```python
from build123d import *

# Parameters (mm, degrees)
F1_DEPTH = 0.91
F3_DEPTH = 5.4
F4_R     = 2.375
F5_DEPTH = 1
F6_R     = 2.375
F7_DEPTH = 3
F9_D     = 2.5
F11_D    = 1


with BuildPart() as f1:
    # F0 (on Top) → F1 (new body, symmetric)
    with BuildSketch(Plane.XY):
        with BuildLine():
            Line((-13.92, -1.75), (-13.92, 1.75))
            ThreePointArc((-13.92, 1.75), (-15.67, 0), (-13.92, -1.75))
        make_face()
        with BuildLine():
            ThreePointArc((-13.92, 1.75), (-12.682563, 1.237437), (-12.17, 0))
            ThreePointArc((-12.17, 0), (-12.682563, -1.237437), (-13.92, -1.75))
            Line((-13.92, -1.75), (0, -2.45))
            Line((0, -2.45), (0, 2.45))
            Line((0, 2.45), (-13.92, 1.75))
        make_face()
        with BuildLine():
            ThreePointArc((-13.92, -1.75), (-12.682563, -1.237437), (-12.17, 0))
            ThreePointArc((-12.17, 0), (-12.682563, 1.237437), (-13.92, 1.75))
            Line((-13.92, 1.75), (-13.92, -1.75))
        make_face()
    extrude(amount=F1_DEPTH, both=True)

    # F2 (on face) → F3 (join)
    with BuildSketch(Plane.XY.offset(0.91)):
        with BuildLine():
            ThreePointArc((-2.509238, -2.323817), (1.24796, -3.184179), (3.42, 0))
            ThreePointArc((3.42, 0), (1.24796, 3.184179), (-2.509238, 2.323817))
            Line((-2.509238, 2.323817), (0, 2.45))
            Line((0, 2.45), (0, -2.45))
            Line((0, -2.45), (-2.509238, -2.323817))
        make_face()
        with BuildLine():
            Line((0, 2.45), (-2.509238, 2.323817))
            ThreePointArc((-2.509238, 2.323817), (-3.42, 0), (-2.509238, -2.323817))
            Line((-2.509238, -2.323817), (0, -2.45))
            Line((0, -2.45), (0, 2.45))
        make_face()
    extrude(amount=-F3_DEPTH)

    # F4 (on face) → F5 (cut)
    with BuildSketch(Plane.XY.offset(0.91)):
        Circle(F4_R)
    extrude(amount=-F5_DEPTH, mode=Mode.SUBTRACT)

    # F6 (on face) → F7 (cut)
    with BuildSketch(Plane(origin=(0, 0, -4.49), x_dir=(1, 0, 0), z_dir=(0, 0, -1))):
        Circle(F6_R)
    extrude(amount=-F7_DEPTH, mode=Mode.SUBTRACT)

    # F9 (through all)
    with Locations(Plane.XY.offset(-0.09)):
        with Locations((0, 0)):
            Hole(F9_D / 2)

    # F11 (through all)
    with Locations(Plane.XY.offset(0.91)):
        with Locations((-14.67, 0), (-12.67, 0), (-10.67, 0), (-8.67, 0), (-6.67, 0), (-4.67, 0)):
            Hole(F11_D / 2)


solid = f1.part
```
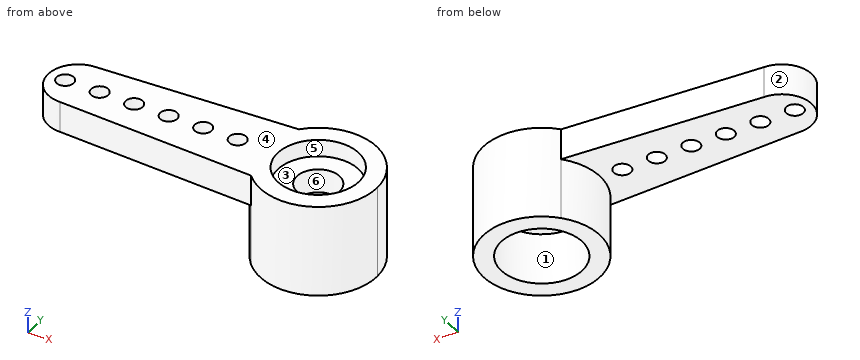
Here's how the part is built. I have some questions about the finished solid (model axes, mm). Face numbers are marked on the shaded views. A direction names the side the tool comes from. Round coordinates to 2 decimals unless told otherwise and drop trailing zeros. Order: outer loops, then holes, each group sorted by start corner. A loop starts at its lowest first (then second) coordinate and runs counter-clockwise, first axis right, second up. Notation, with made-up numbers: (-9, 50) -> (27, 50) arc R21 cw to (27, 67) -> close; hole circle Ø3 at (-2, 81.5). An arc over 180 degrees is marked (long way). Use a Markdown table: item, result. Add a question column.
(1) For pin 1 Ø1.5 at (x, z) = (-13.5, -2) entering from -Y; pin 2 Ø2 at (x, z) = (-13, -0.5) entering from -Y; pin 3 Ø3 at (x, y) = (0, 0) entering from -Z; pin 4 Ø1.4 at (x, y) = (-8.5, 1) entering from -Z, each with a flat end and sliding along its axis, tell me the tip position at first contact or that it passes through.
(2) Suppose I cut it at D-D, the plane x = -2. Please give me the cut outline in (y, z).
(3) If we mould it in two halves opening along X, with no side actions, what happens to the marked faces 1, 2, 3 and 4? For each: released by +X, released by -X, zero draft, split by the parting line, or undercut.
(4) Suppose I cut it at B-B, the plane z = -0.5. Please give me the cut outline in (x, y).
(5) For the marked faces 5 and 6, which set-ups out of +Z, -Z, +X, -X, +Y, -Y let a thin tool reach every point of the face, with its end or its side?
(6) Suppose I cut it at A-A, the plane x = 0. Please give me the cut outline in (y, z) (3 decimals), and give its area (3 significant figures).
(7) Suppose I cut it at C-C, the plane y = -2. Please give me the cut outline in (x, z), and give its area (3 significant figures).
(8) I need wall thicknesses on line 1 along Y through (x, z) = (0, -2.4) (3 decimals); line 2 along X through (y, z) = (1.5, -2); line 3 along X through (y, z) = (1, -1.3). Which ranges of each line are inside material? Lowest first, please.
Verdict:
| question | item | result |
|---|---|---|
| 1 | pin 1 | through |
| 1 | pin 2 | y = -1.85 |
| 1 | pin 3 | z = -1.49 |
| 1 | pin 4 | z = -0.91 |
| 2 | outline | (-2.77, -4.49) -> (-1.28, -4.49) -> (-1.28, -1.49) -> (1.28, -1.49) -> (1.28, -4.49) -> (2.77, -4.49) -> (2.77, 0.91) -> (1.28, 0.91) -> (1.28, -0.09) -> (-1.28, -0.09) -> (-1.28, 0.91) -> (-2.77, 0.91) -> close |
| 3 | face 1 | undercut |
| 3 | face 2 | released by -X |
| 3 | face 3 | undercut |
| 3 | face 4 | zero draft |
| 4 | outline | (-13.92, -1.75) -> (-2.51, -2.32) arc R3.42 ccw (long way) to (-2.51, 2.32) -> (-13.92, 1.75) arc R1.75 ccw to start; hole circle Ø1 at (-14.67, 0); hole circle Ø1 at (-12.67, 0); hole circle Ø1 at (-10.67, 0); hole circle Ø1 at (-8.67, 0); hole circle Ø1 at (-6.67, 0); hole circle Ø1 at (-4.67, 0); hole circle Ø2.5 at (0, 0) |
| 5 | face 5 | +Z |
| 5 | face 6 | +Z, -Z |
| 6 | outline | (-3.42, -4.49) -> (-2.375, -4.49) -> (-2.375, -1.49) -> (-1.25, -1.49) -> (-1.25, -0.09) -> (-2.375, -0.09) -> (-2.375, 0.91) -> (-3.42, 0.91) -> close; (1.25, -1.49) -> (2.375, -1.49) -> (2.375, -4.49) -> (3.42, -4.49) -> (3.42, 0.91) -> (2.375, 0.91) -> (2.375, -0.09) -> (1.25, -0.09) -> close |
| 6 | area | 14.4 mm2 |
| 7 | outline | (-8.95, -0.91) -> (-2.77, -0.91) -> (-2.77, -4.49) -> (-1.28, -4.49) -> (-1.28, -1.49) -> (1.28, -1.49) -> (1.28, -4.49) -> (2.77, -4.49) -> (2.77, 0.91) -> (1.28, 0.91) -> (1.28, -0.09) -> (-1.28, -0.09) -> (-1.28, 0.91) -> (-8.95, 0.91) -> close |
| 7 | area | 31.0 mm2 |
| 8 | line 1 | -3.42 to -2.375, 2.375 to 3.42 |
| 8 | line 2 | -3.07 to -1.84, 1.84 to 3.07 |
| 8 | line 3 | -3.27 to -0.75, 0.75 to 3.27 |
